Can you work these out from the drawing? Everything is in mm from the part's minimum corner. A direction names the side the tool comes from. Coordinates: 2 decimals unless noted, no trailing zeros. Order: outer loops, then holes, each group sorted by start corner. A loop starts at its lowest first (then second) coordinate and runs counter-clockwise, first axis right, second up. Notation, with made-up numbers: (-18, 41) -> (-3, 41) arc R21 cw to (-3, 59) -> close; hole circle Ø6 at (13.25, -5). An arc over 180 degrees is marked (long way). Put each result on its own line as item: value. Start each with the question number.
Q1. We'd pull the mould along X, two halves only. Please class the marked faces 1, 2, 3 and 4: +X half, -X half, draft (parallel to the pull), parting line (faces both ways), or undercut.
Q2. For the marked faces 5, 6 and 7, which set-ups out of +Z, -Z, +X, -X, +Y, -Y let a thin tool reach every point of the face, with its end or its side?
Q3. If we section it at D-D (y = 1.1): Please give me the cut outline in (x, z).
Q4. If we section it at C-C (z = 5.5): Please give me the cut outline in (x, y).
Q5. If we section it at A-A (y = 2.75): Please give me the cut outline in (x, z).
Q6. Will these pins go through, and if not, where does the flat tip stop? pin 1 (3 mm diameter, centred on y = 1, z = 5.5, fed in from -X); pin 2 (0.8 mm diameter, centred on x = 3, y = 3.5, fed in from -Z); pin 3 (2 mm diameter, centred on y = 1.5, z = 7, fed in from +X).
Q7. Please list where these lines run through material, in increasing order: line 1 along Z through (x, y) = (2.15, 2.9); line 2 along Z through (x, y) = (4.85, 2.85); line 3 along Y through (x, z) = (2.8, 6.25).
Q8. If we section it at B-B (x = 3.2): Please give me the cut outline in (y, z).
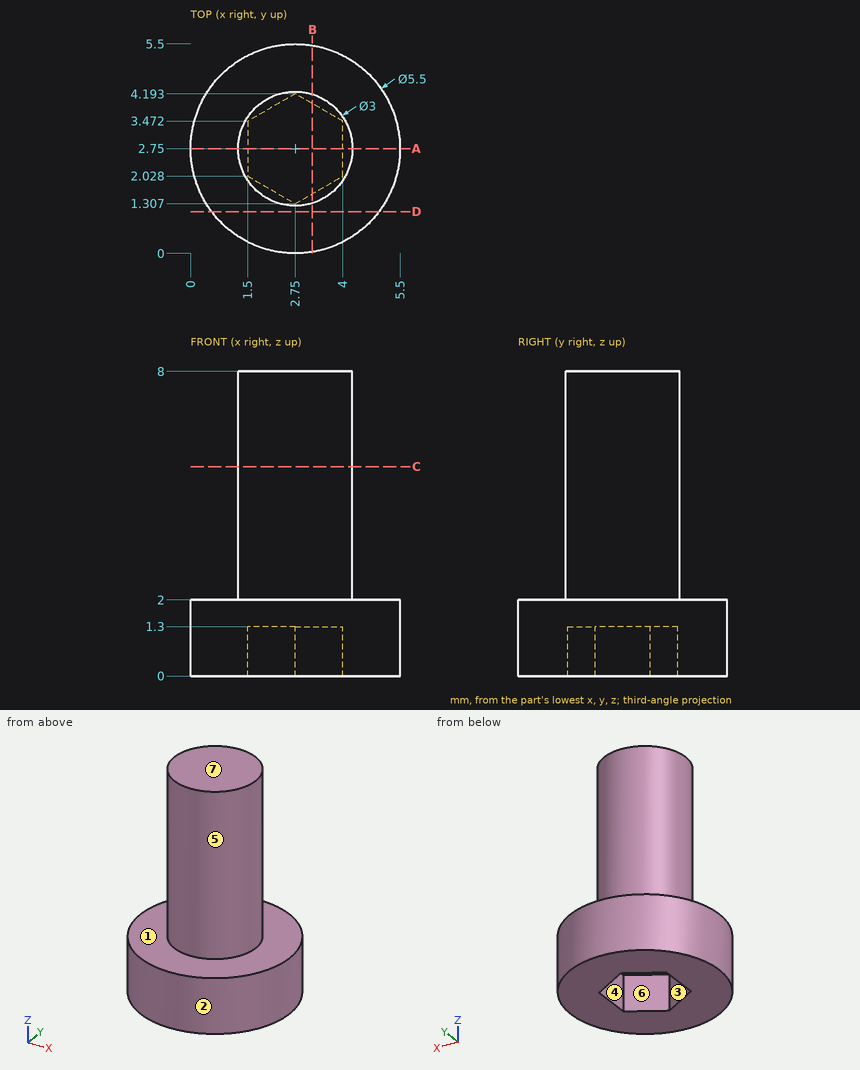
The answers:
1. face 1: draft
1. face 2: parting line
1. face 3: undercut
1. face 4: undercut
2. face 5: +Z
2. face 6: -Z
2. face 7: +Z, +X, -X, +Y, -Y
3. outline: (0.55, 0) -> (4.95, 0) -> (4.95, 2) -> (0.55, 2) -> close
4. outline: circle Ø3 at (2.75, 2.75)
5. outline: (0, 0) -> (1.5, 0) -> (1.5, 1.3) -> (4, 1.3) -> (4, 0) -> (5.5, 0) -> (5.5, 2) -> (4.25, 2) -> (4.25, 8) -> (1.25, 8) -> (1.25, 2) -> (0, 2) -> close
6. pin 1: x = 1.27
6. pin 2: z = 1.3
6. pin 3: x = 4.23
7. line 1: 1.3 to 8
7. line 2: 0 to 2
7. line 3: 1.25 to 4.25
8. outline: (0.04, 0) -> (1.57, 0) -> (1.57, 1.3) -> (3.93, 1.3) -> (3.93, 0) -> (5.46, 0) -> (5.46, 2) -> (4.18, 2) -> (4.18, 8) -> (1.32, 8) -> (1.32, 2) -> (0.04, 2) -> close
